```python
from build123d import *

# Parameters (mm, degrees)
F0_W      = 67.1
F0_H      = 138.3
F1_DEPTH  = 3.55
F2_T      = -2.5
F3_R      = 5
F4_W      = 15.2049176395
F4_H      = 6.8852454424
F5_DEPTH  = 12.5
F7_R      = 5
F8_DEPTH  = 25
F9_W      = 2.0960036782
F9_H      = 22.5108209997
F10_DEPTH = 12.5


with BuildPart() as f1:
    # F0 (on Front) → F1 (new body, symmetric)
    with BuildSketch(Plane.XZ):
        Rectangle(F0_W, F0_H)
    extrude(amount=F1_DEPTH, both=True)

    # F2
    f2_openings = [f1.faces().sort_by_distance(p)[0] for p in [
        (0, -3.55, 0),
    ]]
    offset(amount=F2_T, openings=f2_openings)

    # F3
    f3_edges = [f1.edges().sort_by_distance(p)[0] for p in [
        (-33.55, 0, 69.15),
        (33.55, 0, 69.15),
        (33.55, 0, -69.15),
        (-33.55, 0, -69.15),
    ]]
    fillet(f3_edges, radius=F3_R)

    # F4 (on face) → F5 (cut, symmetric)
    with BuildSketch(Plane.XZ.offset(-1.05)):
        Polygon((12.9098352045, 53.504101932), (12.9098352045, 60.3893473744), (28.114752844, 60.3893473744), (28.114752844, 53.504101932), (31.05, 53.504101932), (31.05, 66.65), (0, 66.65), (0, 53.504101932), align=None)
        with Locations((20.5122940242, 56.9467246532)):
            Rectangle(F4_W, F4_H)
    extrude(amount=F5_DEPTH, both=True, mode=Mode.SUBTRACT)

    # F7
    f7_edges = [f1.edges().sort_by_distance(p)[0] for p in [
        (0, 2.3, 53.504102),
        (0, 2.3, 66.65),
        (31.05, 0, 66.65),
        (31.05, 2.3, 53.504102),
    ]]
    fillet(f7_edges, radius=F7_R)

    # F6 (on face) → F8 (cut)
    with BuildSketch(Plane.XY.offset(-66.65)):
        Polygon((5.7946089791, 1.05), (-30.1529895514, 1.05), (-30.1529895514, -3.55), (31.05, -3.55), (31.05, 1.05), align=None)
    extrude(amount=-F8_DEPTH, mode=Mode.SUBTRACT)

    # F9 (on face) → F10 (cut, symmetric)
    with BuildSketch(Plane(origin=(-33.55, 0, 0), x_dir=(0, -1, 0), z_dir=(-1, 0, 0))):
        with Locations((0.850938115, 39.116631262)):
            Rectangle(F9_W, F9_H)
    extrude(amount=F10_DEPTH, both=True, mode=Mode.SUBTRACT)


solid = f1.part
```
Build history of the part. All positions in model axes, mm. A direction names the side the tool comes from. Round coordinates to 2 decimals unless told otherwise and drop trailing zeros. Loops run counter-clockwise (first coordinate to the right, second up) from the corner with the lowest first, then second, coordinate; pieces in that order, holes last.
Item 1: Saw through at D-D (x = -8.5). List the corners of the cut face in (y, z), then the cut area to 3 significant figures.
Item 2: Saw through at B-B (x = 16). List the corners of the cut face in (y, z), then the cut area to 3 significant figures.
Item 3: Saw through at C-C (z = 15). List the corners of the cut face in (x, y), then the cut area to 3 significant figures.
Item 4: Drill centre lines: line 1 along X through (y, z) = (-2.25, -31.5); line 2 along Z through (x, y) = (18.5, 2.25). Where is each one in solid material? Low to high.
Item 5: Which spindle directions (+Z, -Z, +X, -X, +Y, -Y) get a long thin tool onto all of the face, cutting with end or side? Do faces 1 (the face through (15, 2, 53.504)), 2 (the face through (-2, -1, 66.65)), 3 (the face through (-32, 0.197, 39)). Say none if no direction does.
Item 6: Pin check, flat tips, straight feed: P1, Ø2, axis at x = -0.5, z = -55, coming from the -Y side; P2, Ø1.7, axis at x = -32.5, y = -0.5, coming from the +Z side; P3, Ø0.7, axis at y = -1, z = -68, coming from the +X side. Stop position of each tip, or through.
Item 7: Saw through at A-A (z = 30.5). List the corners of the cut face in (x, y).
Item 8: Two-plate mould, pull along Y, no slides. Class faces 4 (the face through (-32, -1.899, 39)), 5 (the face through (0, 3.55, 1)), 6 (the face through (1.504, 2.318, 54.93)): released by +Y, released by -Y, zero draft, split by the parting line, or undercut.
Worked answers:
1. outline: (-3.55, 66.65) - (1.05, 66.65) - (1.05, -69.15) - (3.55, -69.15) - (3.55, 69.15) - (-3.55, 69.15) - close
1. area: 357 mm2
2. outline: (-3.55, 66.65) - (3.55, 66.65) - (3.55, 69.15) - (-3.55, 69.15) - close; (1.05, -69.15) - (3.55, -69.15) - (3.55, 53.5) - (1.05, 53.5) - close
2. area: 324 mm2
3. outline: (-33.55, -3.55) - (-31.05, -3.55) - (-31.05, 1.05) - (31.05, 1.05) - (31.05, -3.55) - (33.55, -3.55) - (33.55, 3.55) - (-33.55, 3.55) - close
3. area: 191 mm2
4. line 1: x = -33.55 to -31.05, 31.05 to 33.55
4. line 2: z = -69.15 to 53.5, 66.65 to 69.15
5. face 1: +Y, -Y
5. face 2: -Y
5. face 3: -X
6. P1: stops at y = 1.05
6. P2: stops at z = 68.07
6. P3: stops at x = 32.12
7. outline: (-33.55, -3.55) - (-31.05, -3.55) - (-31.05, -1.9) - (-33.55, -1.9) - close; (-33.55, 0.2) - (-31.05, 0.2) - (-31.05, 1.05) - (31.05, 1.05) - (31.05, -3.55) - (33.55, -3.55) - (33.55, 3.55) - (-33.55, 3.55) - close
8. face 4: undercut
8. face 5: released by +Y
8. face 6: zero draft
